Can you work these out from the model? Positions are in its coordinate system, mm. Face numbers are marked on the shaded views. A direction names the side the tool comes from. Coordinates: 2 decimals unless noted, no trailing zeros. Write each loop counter-clockwise with the first axis right and the second up, starting at its lowest first coordinate (ties: lowest second). Pieces come first, ordered by that corner, then holes. Notation, with made-up numbers: (23.5, 19) - (29.5, 19) arc R13 cw to (29.5, 41) - close; hole circle Ø4 at (58, 85). An arc over 180 degrees is marked (long way). Use one line per item in the form item = value. Start each with the question number.
(1) If we section it at A-A on x = 0: Please give me the cut outline in (y, z).
(2) For pin 1 Ø5 at (x, z) = (-30.5, 2) entering from +Y; pin 2 Ø5 at (x, z) = (-30, 4) entering from -Y; pin 3 Ø1.5 at (x, z) = (-1, 3.5) entering from -Y, each with a flat end and sliding along its axis, tell me the tip position at first contact or that it passes through.
(3) On a 3-axis mill with a long thin cutter (end or side, diameter ignored), from which of +Z, -Z, +X, -X, +Y, -Y can I reach the whole of each face in a straight line? I mean the marked faces 4, 5 and 6. Say none if no direction works.
(4) If we section it at C-C on x = -44: Please give me the cut outline in (y, z).
(5) If I drill on probe 1 along Y at (x, z) = (4.5, 7.5); probe 2 along X at (y, z) = (41, 9.5); probe 3 along X at (y, z) = (13, 4.25), over which ranges is the centre line in solid material (lowest first)? Write a range as from..to.
(6) Thinking about a two-plate mould opening in X: for the marked faces 1, 2 and 3, which applies, pulls with the +X half, pulls with the -X half, needs draft (parallel to the pull), parting line crosses it, or undercut?
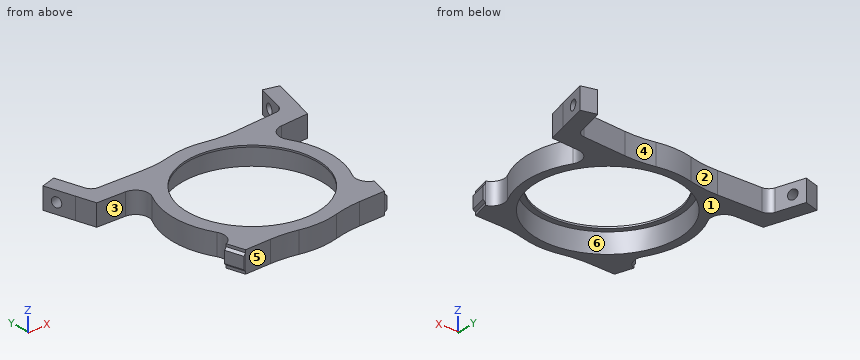
```python
from build123d import *

# Parameters (mm, degrees)
SKIZZE1_R                       = 32.75
AUFSATZ_LINEAR_AUSTRAGEN1_DEPTH = 10
AUFSATZ_LINEAR_START            = -0.8
SKIZZE2_R                       = 32.75
SKIZZE2_R_2                     = 30.25
AUFSATZ_LINEAR_AUSTRAGEN2_DEPTH = 0.8
SKIZZE5_R                       = 2.25
SCHNITT_LINEAR_AUSTRAGEN1_DEPTH = 10
VERRUNDUNG1_R                   = 50
VERRUNDUNG2_R                   = 6
VERRUNDUNG3_R                   = 4
AUFSATZ_LINEAR_AUSTRAGEN3_DEPTH = 8.306468


with BuildPart() as part:
    # Skizze1 → Aufsatz-Linear austragen1 (new body)
    with BuildSketch(Plane.XY):
        with BuildLine():
            Line((-13.635878322, -34.12660725), (-33.089645956, -34.12660725))
            Line((-33.089645956, -34.12660725), (-35.325135331, -26.12660725))
            Line((-35.325135331, -26.12660725), (-25.844978112, -26.12660725))
            ThreePointArc((-25.844978112, -26.12660725), (-36.75, 0), (-25.844978112, 26.12660725))
            Line((-25.844978112, 26.12660725), (-50.235580292, 27.232429468))
            Line((-50.235580292, 27.232429468), (-52.656417654, 35.895722216))
            Line((-52.656417654, 35.895722216), (-56.424186432, 49.379190555))
            Line((-56.424186432, 49.379190555), (-49.682452262, 51.263074944))
            Line((-49.682452262, 51.263074944), (-45.294995525, 35.561969729))
            Line((-45.294995525, 35.561969729), (-13.635878322, 34.12660725))
            ThreePointArc((-13.635878322, 34.12660725), (0, 36.75), (13.635878322, 34.12660725))
            Line((13.635878322, 34.12660725), (45.294995525, 35.561969729))
            Line((45.294995525, 35.561969729), (49.682452262, 51.263074944))
            Line((49.682452262, 51.263074944), (56.424186432, 49.379190555))
            Line((56.424186432, 49.379190555), (52.656417654, 35.895722216))
            Line((52.656417654, 35.895722216), (50.235580292, 27.232429468))
            Line((50.235580292, 27.232429468), (25.844978112, 26.12660725))
            ThreePointArc((25.844978112, 26.12660725), (36.75, 0), (25.844978112, -26.12660725))
            Line((25.844978112, -26.12660725), (35.325135331, -26.12660725))
            Line((35.325135331, -26.12660725), (33.089645956, -34.12660725))
            Line((33.089645956, -34.12660725), (13.635878322, -34.12660725))
            ThreePointArc((13.635878322, -34.12660725), (0, -36.75), (-13.635878322, -34.12660725))
        make_face()
        Circle(SKIZZE1_R, mode=Mode.SUBTRACT)
    extrude(amount=AUFSATZ_LINEAR_AUSTRAGEN1_DEPTH)

    # Skizze2 → Aufsatz-Linear austragen2 (add)
    with BuildSketch(Plane.XY.offset(10).offset(AUFSATZ_LINEAR_START)):
        Circle(SKIZZE2_R)
        Circle(SKIZZE2_R_2, mode=Mode.SUBTRACT)
    extrude(amount=AUFSATZ_LINEAR_AUSTRAGEN2_DEPTH)

    # Skizze5 → Schnitt-Linear austragen1 (cut)
    with BuildSketch(Plane(origin=(32.796772797, -9.164604643, 0), x_dir=(0, 0, 1), z_dir=(-0.9631048813334842, 0.2691263412444341, 0))):
        with Locations(Location((5, 56.94978804, 0), (0, 0, 270))):
            Circle(SKIZZE5_R)
    schnitt_linear_austragen1 = extrude(amount=-SCHNITT_LINEAR_AUSTRAGEN1_DEPTH, mode=Mode.SUBTRACT)

    # Spiegeln1: Schnitt-Linear austragen1 across plane
    add(schnitt_linear_austragen1.mirror(Plane(origin=(0, 0, 0), x_dir=(0, 0, 1), z_dir=(1, 0, 0))), mode=Mode.SUBTRACT)

    # Verrundung1
    verrundung1_edges = [part.edges().sort_by_distance(p)[0] for p in [
        (13.635878322, 34.12660725, 5),
        (13.635878322, -34.12660725, 5),
        (-13.635878322, -34.12660725, 5),
        (-13.635878322, 34.12660725, 5),
    ]]
    fillet(verrundung1_edges, radius=VERRUNDUNG1_R)

    # Verrundung2
    # the kernel refuses this fillet: 6 mm, written as the material it adds along each edge
    with BuildSketch(Plane(origin=(-25.844978112, -26.12660725, 0), x_dir=(-1, 0, 0), z_dir=(0, 0, 1))) as verrundung2_piece_1:
        with BuildLine():
            CenterArc((11.651069987, -5.593490659), VERRUNDUNG2_R, 111.211936516, 97.493506366)
            Line((6.388466745, -8.475331584), (6.283214681, -8.532968403))
            ThreePointArc((6.283214681, -8.532968403), (3.405977683, -4.078058883), (-0.084391765, -0.085311371))
            Line((-0.084391765, -0.085311371), (0, 0.12))
            ThreePointArc((0, 0.12), (4.74007861, 0.12), (9.436738964, 0.111869813))
            Line((9.436738964, 0.111869813), (9.48015722, 0))
        make_face()
    extrude(amount=10)
    with BuildSketch(Plane(origin=(25.844978112, -26.12660725, 0), x_dir=(1, 0, 0), z_dir=(0, 0, 1))) as verrundung2_piece_2:
        with BuildLine():
            CenterArc((11.651069987, 5.593490659), VERRUNDUNG2_R, 151.294557118, 97.493506366)
            Line((6.388466745, 8.475331584), (6.283214681, 8.532968403))
            ThreePointArc((6.283214681, 8.532968403), (3.405977683, 4.078058883), (-0.084391765, 0.085311371))
            Line((-0.084391765, 0.085311371), (0, -0.12))
            ThreePointArc((0, -0.12), (4.74007861, -0.12), (9.436738964, -0.111869813))
            Line((9.436738964, -0.111869813), (9.48015722, 0))
        make_face()
    extrude(amount=10)
    with BuildSketch(Plane(origin=(25.844978112, 26.12660725, 0), x_dir=(0.603126946859045, -0.7976452130944475, 0), z_dir=(0, 0, 1))) as verrundung2_piece_3:
        with BuildLine():
            CenterArc((11.361383868, 5.938413704), VERRUNDUNG2_R, 145.501722428, 116.281978681)
            Line((6.416524574, 9.336702474), (6.317627388, 9.40466825))
            Line((6.317627388, 9.40466825), (-0.098897186, 0.067965775))
            Line((-0.098897186, 0.067965775), (0.017149259, -0.118768274))
            ThreePointArc((0.017149259, -0.118768274), (5.251960467, 0.257216064), (10.486771676, -0.118768274))
            Line((10.486771676, -0.118768274), (10.503920934, 0))
        make_face()
    extrude(amount=10)
    with BuildSketch(Plane(origin=(-25.844978112, 26.12660725, 0), x_dir=(-0.6031269468590452, -0.7976452130944475, 0), z_dir=(0, 0, 1))) as verrundung2_piece_4:
        with BuildLine():
            CenterArc((11.361383868, -5.938413704), VERRUNDUNG2_R, 98.216298891, 116.281978681)
            Line((6.416524574, -9.336702474), (6.317627388, -9.40466825))
            Line((6.317627388, -9.40466825), (-0.098897186, -0.067965775))
            Line((-0.098897186, -0.067965775), (0.017149259, 0.118768274))
            ThreePointArc((0.017149259, 0.118768274), (5.251960467, -0.257216064), (10.486771676, 0.118768274))
            Line((10.486771676, 0.118768274), (10.503920934, 0))
        make_face()
    extrude(amount=10)

    # Verrundung3
    verrundung3_edges = [part.edges().sort_by_distance(p)[0] for p in [
        (45.294995525, 35.561969729, 5),
        (-45.294995525, 35.561969729, 5),
    ]]
    fillet(verrundung3_edges, radius=VERRUNDUNG3_R)

    # Skizze6 → Aufsatz-Linear austragen3 (add)
    with BuildSketch(Plane(origin=(6.448861011, -23.078118218, 0), x_dir=(0, 0, -1), z_dir=(-0.26912634124443396, 0.9631048813334842, 0))):
        Polygon((-8.75, 41.05316849), (-7.75, 42.05316849), (-2.25, 42.05316849), (-1.25, 41.05316849), align=None)
    aufsatz_linear_austragen3 = extrude(amount=AUFSATZ_LINEAR_AUSTRAGEN3_DEPTH)

    # Spiegeln2: Aufsatz-Linear austragen3 across plane
    add(aufsatz_linear_austragen3.mirror(Plane(origin=(0, 0, 0), x_dir=(0, 0, 1), z_dir=(1, 0, 0))))


solid = part.part
```
Reported:
q1.outline = (-36.75, 0) - (-32.75, 0) - (-32.75, 9.2) - (-30.25, 9.2) - (-30.25, 10) - (-36.75, 10) - close; (30.25, 9.2) - (32.75, 9.2) - (32.75, 0) - (36.75, 0) - (36.75, 10) - (30.25, 10) - close
q2.pin_1 = 35
q2.pin_2 = -34.13
q2.pin_3 = -36.75
q3.face_4 = +Z, -Z, +Y
q3.face_5 = +Z, -Z, -Y
q3.face_6 = -Z
q4.outline = (26.95, 0) - (35.84, 0) - (35.84, 10) - (26.95, 10) - close
q5.probe_1 = -36.47..-32.44, 32.44..36.47
q5.probe_2 = -54.08..-46.81, 46.81..54.08
q5.probe_3 = -34.37..-30.06, 30.06..34.37
q6.face_1 = needs draft
q6.face_2 = undercut
q6.face_3 = pulls with the -X half
